from build123d import *

# Parameters (mm, degrees)
SKETCH_1_R           = 1
EXTRUDE_1_DEPTH      = 3
EXTRUDE_2_DEPTH      = 2
EXTRUDE_2_DEPTH_BACK = 5
FILLET_START         = -3
FILLET_3_DEPTH       = 9
FILLET_4_R           = 5
CUT_EXTRUDE_2_DEPTH  = 2
CUT_EXTRUDE_3_DEPTH  = 2


with BuildPart() as part:
    # 草图1 → 凸台-拉伸1 (new body)
    with BuildSketch(Plane.XY):
        with BuildLine():
            Line((-5, 0), (-5, -18.11131196))
            Line((-5, -18.11131196), (5, -18.11131196))
            Line((5, -18.11131196), (5, 0))
            ThreePointArc((5, 0), (0, 5), (-5, 0))
        make_face()
        Circle(SKETCH_1_R, mode=Mode.SUBTRACT)
    extrude(amount=EXTRUDE_1_DEPTH)

    # 草图2 → 凸台-拉伸2 (add, two sides: drawn at the far end of the back side and taken through both)
    with BuildSketch(Plane.XY.offset(3).offset(-EXTRUDE_2_DEPTH_BACK)):
        with BuildLine():
            Line((5, -21.0685844), (5, -18.11131196))
            Line((5, -18.11131196), (-5, -18.11131196))
            Line((-5, -18.11131196), (-5, -21.0685844))
            Line((-5, -21.0685844), (-5, -23.814982117))
            Line((-5, -23.814982117), (-2.964275547, -23.744594918))
            add(Edge.make_bspline(
                [(3.626985758, -47.647589684), (-16.682654634, -40.9110727), (-18.879741736, -32.943407778), (-2.964275547, -23.744594918)],
                knots=[0, 0, 0, 0, 0.912623114, 0.912623114, 0.912623114, 0.912623114], degree=3))
            Line((3.626985758, -47.647589684), (3.626985758, -23.516695498))
            Line((3.626985758, -23.516695498), (5.09467917, -23.465948537))
            Line((5.09467917, -23.465948537), (5, -21.0685844))
        make_face()
        with BuildLine():
            add(Edge.make_bspline(
                [(0, -41.401376639), (-15.873118036, -34.591902926), (0, -27.782429212)],
                knots=[0, 0, 0, 1, 1, 1], degree=2))
            Line((0, -27.782429212), (0, -41.401376639))
        make_face(mode=Mode.SUBTRACT)
    extrude(amount=EXTRUDE_2_DEPTH + EXTRUDE_2_DEPTH_BACK)

    # 圆角3: read off the stored shape, not the designer's step
    # 圆角3 outline → 圆角3 (cut)
    with BuildSketch(Plane.XY.offset(FILLET_START)):
        with BuildLine():
            Line((5.09467917, -23.465948537), (5.018307469, -21.532146448))
            ThreePointArc((5.018307469, -21.532146448), (4.657500154, -22.759179091), (3.626985758, -23.516695498))
            Line((3.626985758, -23.516695498), (5.09467917, -23.465948537))
        make_face()
        with BuildLine():
            Line((-5, -23.814982117), (-2.964275547, -23.744594918))
            ThreePointArc((-2.964275547, -23.744594918), (-4.401526149, -23.171702163), (-5, -21.744914003))
            Line((-5, -21.744914003), (-5, -23.814982117))
        make_face()
        with BuildLine():
            Line((3.626985758, -47.647589684), (3.626985758, -44.832103607))
            ThreePointArc((3.626985758, -44.832103607), (2.771627596, -46.472163076), (0.937190695, -46.709384292))
            add(Edge.make_bspline(
                [(3.626985758, -47.647589684), (2.692000341, -47.337463802), (1.795401987, -47.024728671), (0.937190695, -46.709384292)],
                knots=[0, 0, 0, 0, 0.042014004, 0.042014004, 0.042014004, 0.042014004], degree=3))
        make_face()
    extrude(amount=FILLET_3_DEPTH, mode=Mode.SUBTRACT)

    # 圆角4
    fillet_4_edges = [part.edges().sort_by_distance(p)[0] for p in [
        (-2.964275547, -23.744594918, 0.5),
    ]]
    fillet(fillet_4_edges, radius=FILLET_4_R)

    # 草图6 → 切除-拉伸2 (cut)
    with BuildSketch(Plane.XY.offset(5)):
        with BuildLine():
            Line((3.626985758, -21.269208488), (3.626985758, -25.801560292))
            Line((3.626985758, -25.801560292), (5, -25.801560292))
            Line((5, -25.801560292), (5, -18.11131196))
            Line((5, -18.11131196), (-5, -18.11131196))
            Line((-5, -18.11131196), (-5, -21.269208488))
            Line((-5, -21.269208488), (-7.053376084, -26.364298767))
            add(Edge.make_bspline(
                [(3.626985758, -21.269208488), (-2.623871875, -22.388888024), (-7.053376084, -26.364298767)],
                knots=[0, 0, 0, 1, 1, 1], degree=2))
        make_face()
    extrude(amount=-CUT_EXTRUDE_2_DEPTH, mode=Mode.SUBTRACT)

    # 草图7 → 切除-拉伸3 (cut)
    with BuildSketch(Plane(origin=(0, 0, -2), x_dir=(-1, 0, 0), z_dir=(0, 0, -1))):
        with BuildLine():
            Line((-3.626985758, -21.004340975), (-3.626985758, -25.801560292))
            Line((-3.626985758, -25.801560292), (-5, -25.801560292))
            Line((-5, -25.801560292), (-5, -18.11131196))
            Line((-5, -18.11131196), (7.053376084, -18.11131196))
            Line((7.053376084, -18.11131196), (7.053376084, -26.364298767))
            add(Edge.make_bspline(
                [(-3.626985758, -21.004340975), (2.577596391, -22.360926345), (7.053376084, -26.364298767)],
                knots=[0, 0, 0, 1, 1, 1], degree=2))
        make_face()
    extrude(amount=-CUT_EXTRUDE_3_DEPTH, mode=Mode.SUBTRACT)


solid = part.part
Could you check a few things on this model? Use its own coordinates, in mm. A direction names the side the tool comes from. Give positions to 0.01 mm unless a question says otherwise; leave off trailing zeros. Order: outer loops, then holes, each group sorted by start corner. A loop starts at its lowest first (then second) coordinate and runs counter-clockwise, first axis right, second up. Notation, with made-up numbers: (77.25, 14.25) - (106.25, 14.25) arc R33 cw to (106.25, 50.25) - close; hole circle Ø6 at (-9.75, 46). An arc over 180 degrees is marked (long way). One line per item, written item: value. Start each with the question number.
1. Thinking about a two-plate mould opening in Y: for faces 3 (the face through (2.79, -46.46, 1.45)), 4 (the face through (3.627, -33, 2)), 5 (the face through (0, -34, 1)), which applies, +Y half, -Y half, draft (parallel to the pull), parting line (faces both ways), or undercut?
2. For faces 1 (the face through (0, 5, 1)), 2 (the face through (-5, -11, 1)), which set-ups out of +Z, -Z, +X, -X, +Y, -Y let a thin tool reach every point of the face, with its end or its side?
3. Imagine slicing it at A-A on z = 4. Give the number of separate pieces and of enclosed holes in the cut face, plus the area to 3 significant figures.
4. For P1, Ø3.5, axis at y = -7.5, z = 2, coming from the +X side; P2, Ø1.5, axis at y = -37, z = -0.5, coming from the -X side; P3, Ø4, axis at x = -1, y = -9.5, coming from the +Z side; P4, Ø1.6, axis at x = 0, y = 0, coming from the +Z side, each with a flat end and sliding along its axis, tell me the tip position at first contact or that it passes through.
5. Imagine slicing it at B-B on y = -17. List the corners of the cut face in (x, z) for me, plus the area to 3 significant figures.
6. Imagine slicing it at C-C on y = 2.5. List the corners of the cut face in (x, z) for me.
7. If I drill on probe 1 along Y at (x, z) = (-0.75, 1.5); probe 2 along Y at (x, z) = (-7.5, 2.5); probe 3 along X at (y, z) = (-16.5, 0.75), over which ranges is the centre line in solid material (lowest first)?
Values:
1. face 3: -Y half
1. face 4: draft
1. face 5: undercut
2. face 1: +Z, -Z, +Y
2. face 2: +Z, -Z, -X, +Y
3. separate pieces: 2
3. enclosed holes: 1
3. area: 236 mm²
4. P1: x = 5
4. P2: x = -13.34
4. P3: z = 3
4. P4: through
5. outline: (-5, 0) - (5, 0) - (5, 3) - (-5, 3) - close
5. area: 30.0 mm²
6. outline: (-4.33, 0) - (4.33, 0) - (4.33, 3) - (-4.33, 3) - close
7. probe 1: -46.07 to -41.07, -28.11 to -0.66, 0.66 to 4.94
7. probe 2: -42.81 to -36.19, -32.99 to -26.69
7. probe 3: -5 to 5
